Can you work these out from the model? Positions are in its coordinate system, mm. Give positions to 0.01 mm unless a question says otherwise; leave off trailing zeros. Write each loop counter-clockwise with the first axis right and the second up, starting at its lowest first coordinate (ties: lowest second). Pieces come first, ordered by that corner, then holes.
1. Suppose I cut it at A-A (y = -2). Please give me the cut outline in (x, z), and give its area (3 significant figures).
2. Suppose I cut it at C-C (x = -187). Please give me the cut outline in (y, z), and give its area (3 significant figures).
3. Suppose I cut it at B-B (z = 3). Give the number of separate pieces and of enclosed holes in the cut face, and give its area (3 significant figures).
4. If I drill on probe 1 along X at (y, z) = (14, 4.6); probe 2 along Y at (x, z) = (227, 2.4), over which ranges is the centre line in solid material (lowest first)?
5. I'm going to push flat-ended pins straight in: pin 1 (1.8 mm diameter, centred on x = -234.5, z = 3, fed in from -Y); pin 2 (1.8 mm diameter, centred on y = -29.5, z = 2, fed in from +X). Where does each tip first touch, or does it pass through?
```python
from build123d import *

# Parameters (mm, degrees)
CROQUIS1_W              = 510
CROQUIS1_H              = 55
SALIENTE_EXTRUIR1_DEPTH = 6
CORTAR_EXTRUIR1_REACH   = 8
CROQUIS2_W              = 5.8
CROQUIS2_H              = 29.8
CROQUIS3_W              = 30
CROQUIS3_H              = 6
SALIENTE_EXTRUIR2_DEPTH = 6


with BuildPart() as part:
    # Croquis1 → Saliente-Extruir1 (new body)
    with BuildSketch(Plane.XY):
        Rectangle(CROQUIS1_W, CROQUIS1_H)
    extrude(amount=SALIENTE_EXTRUIR1_DEPTH)

    # Croquis2 → Cortar-Extruir1 (cut, up to next)
    with BuildSketch(Plane.XY.offset(6), mode=Mode.PRIVATE) as cortar_extruir1_sk1:
        with Locations((-246.1, 0)):
            Rectangle(CROQUIS2_W, CROQUIS2_H)
    cortar_extruir1_tool1 = extrude(cortar_extruir1_sk1.sketch, amount=-CORTAR_EXTRUIR1_REACH, mode=Mode.PRIVATE) & part.part
    add(cortar_extruir1_tool1.solids().sort_by_distance((-246.1, 0, 6))[0], mode=Mode.SUBTRACT)
    # Croquis2 → Cortar-Extruir1 (cut, up to next)
    with BuildSketch(Plane.XY.offset(6), mode=Mode.PRIVATE) as cortar_extruir1_sk2:
        with Locations((246.1, 0)):
            Rectangle(CROQUIS2_W, CROQUIS2_H)
    cortar_extruir1_tool2 = extrude(cortar_extruir1_sk2.sketch, amount=-CORTAR_EXTRUIR1_REACH, mode=Mode.PRIVATE) & part.part
    add(cortar_extruir1_tool2.solids().sort_by_distance((246.1, 0, 6))[0], mode=Mode.SUBTRACT)

    # Croquis3 → Saliente-Extruir2 (add)
    with BuildSketch(Plane.XZ.offset(27.5)):
        with Locations((0, 3)):
            Rectangle(CROQUIS3_W, CROQUIS3_H)
        with Locations((105, 3)):
            Rectangle(CROQUIS3_W, CROQUIS3_H)
        with Locations((210, 3)):
            Rectangle(CROQUIS3_W, CROQUIS3_H)
        with Locations((-105, 3)):
            Rectangle(CROQUIS3_W, CROQUIS3_H)
        with Locations((-210, 3)):
            Rectangle(CROQUIS3_W, CROQUIS3_H)
    extrude(amount=SALIENTE_EXTRUIR2_DEPTH)


solid = part.part
```
Checks:
1. outline: (-255, 0) - (-249, 0) - (-249, 6) - (-255, 6) - close; (-243.2, 0) - (243.2, 0) - (243.2, 6) - (-243.2, 6) - close; (249, 0) - (255, 0) - (255, 6) - (249, 6) - close
1. area: 2,990 mm2
2. outline: (-27.5, 0) - (27.5, 0) - (27.5, 6) - (-27.5, 6) - close
2. area: 330 mm2
3. separate pieces: 1
3. enclosed holes: 2
3. area: 28,600 mm2
4. probe 1: x = -255 to -249, -243.2 to 243.2, 249 to 255
4. probe 2: y = -27.5 to 27.5
5. pin 1: stops at y = -27.5
5. pin 2: stops at x = 225
